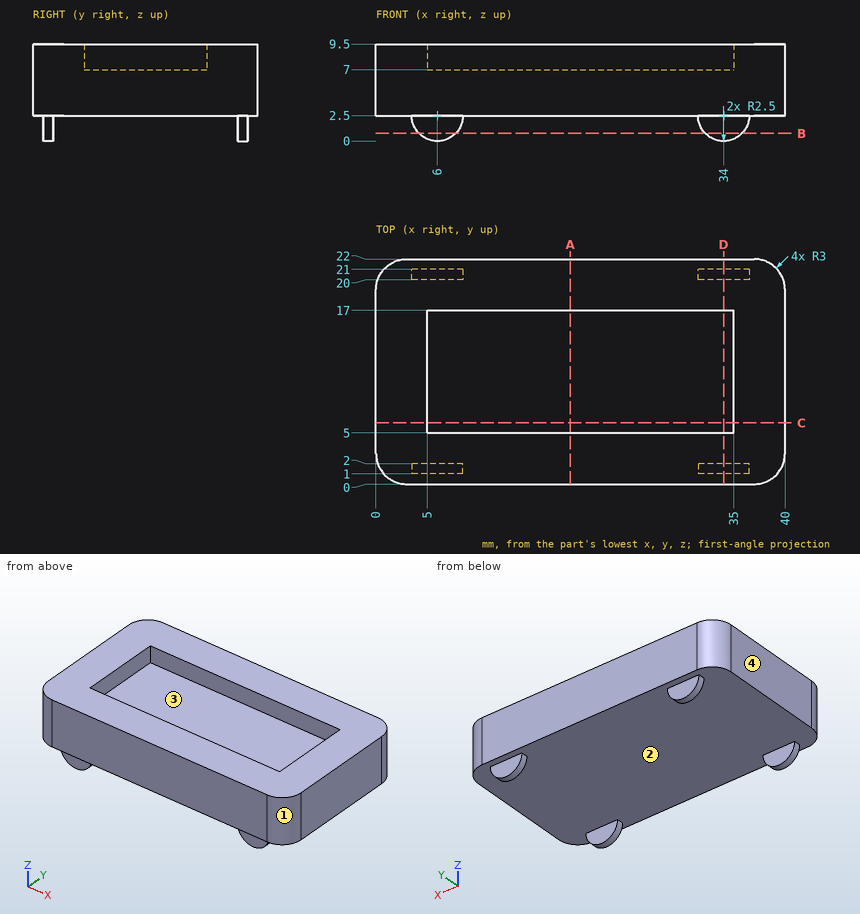
Geometry: see drawing. Coordinates: mm, zero at the bounding-box minimum. Coordinates: 2 decimals unless noted, no trailing zeros. Loops run counter-clockwise (first coordinate to the right, second up) from the corner with the lowest first, then second, coordinate; pieces in that order, holes last. Notation, with made-up numbers: (67, 45) - (74, 45) arc R21 cw to (74, 75) - close; hole circle Ø9 at (46.25, -13). An arc over 180 degrees is marked (long way). Answer as CSV lines item,"result".
1. Section D-D (x = 34). Return loops of the section in (y, z), then the cut area to 3 significant figures.
Established:
outline,"(0, 2.5) - (1, 2.5) - (1, 0) - (2, 0) - (2, 2.5) - (20, 2.5) - (20, 0) - (21, 0) - (21, 2.5) - (22, 2.5) - (22, 9.5) - (17, 9.5) - (17, 7) - (5, 7) - (5, 9.5) - (0, 9.5) - close"
area,"129 mm2"
2. Contact query for flat-ended pins moving along their axis: pin 1 (0.8 mm diameter, centred on x = 33, z = 1.5, fed in from -Y); pin 2 (6 mm diameter, centred on x = 23, y = 9, fed in from +Z); pin 3 (2 mm diameter, centred on x = 5.5, z = 2, fed in from +Y); pin 4 (5 mm diameter, centred on x = 11.5, y = 13.5, fed in from -Z). Output: stop coordinate, or through.
Established:
pin 1,"stops at y = 1"
pin 2,"stops at z = 7"
pin 3,"stops at y = 22"
pin 4,"stops at z = 2.5"
3. Ray query, line 1 (X direction, y = 6.5, z = 8.5); line 2 (Y direction, x = 11, z = 7.75); line 3 (Z direction, x = 38.5, y = 12.5). Return the intervals inside material, ascending.
Established:
line 1,"x = 0 to 5, 35 to 40"
line 2,"y = 0 to 5, 17 to 22"
line 3,"z = 2.5 to 9.5"
4. Mould query, pull axis Y, two halves, no side actions, for the marked faces 1, 2, 3 and 4. Classes: released by +Y, released by -Y, zero draft, split by the parting line, or undercut.
Established:
face 1,"released by -Y"
face 2,"undercut"
face 3,"undercut"
face 4,"zero draft"
5. Section A-A (x = 19). Return loops of the section in (y, z).
Established:
outline,"(0, 2.5) - (22, 2.5) - (22, 9.5) - (17, 9.5) - (17, 7) - (5, 7) - (5, 9.5) - (0, 9.5) - close"
6. Section C-C (y = 6). Return loops of the section in (x, z), then the cut area to 3 significant figures.
Established:
outline,"(0, 2.5) - (40, 2.5) - (40, 9.5) - (35, 9.5) - (35, 7) - (5, 7) - (5, 9.5) - (0, 9.5) - close"
area,"205 mm2"
7. Section B-B (z = 0.75). Return loops of the section in (x, y), then the cut area to 3 significant figures.
Established:
outline,"(4.21, 1) - (7.79, 1) - (7.79, 2) - (4.21, 2) - close; (4.21, 20) - (7.79, 20) - (7.79, 21) - (4.21, 21) - close; (32.21, 1) - (35.79, 1) - (35.79, 2) - (32.21, 2) - close; (32.21, 20) - (35.79, 20) - (35.79, 21) - (32.21, 21) - close"
area,"14.3 mm2"
